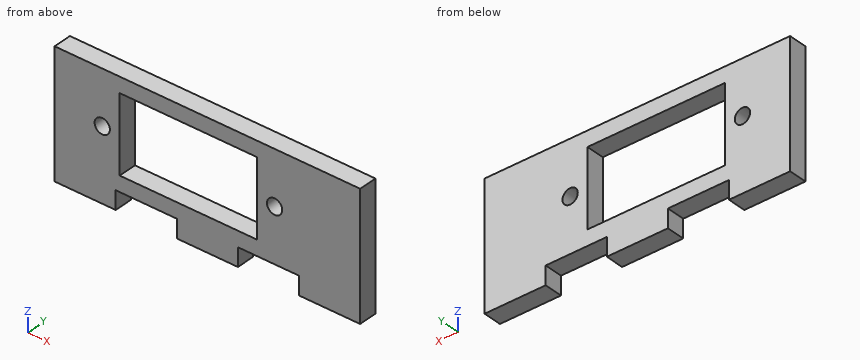
from build123d import *

# Parameters (mm, degrees)
CROQUIS1_R              = 1.25
CROQUIS1_W              = 22.5
CROQUIS1_H              = 12.5
CROQUIS1_W_2            = 10
CROQUIS1_H_2            = 3
SALIENTE_EXTRUIR1_DEPTH = 3


with BuildPart() as part:
    # Croquis1 → Saliente-Extruir1 (new body)
    # profile 1 of 4: a face of its own
    with BuildSketch(Plane(origin=(0, 0, 0), x_dir=(1, 0, 0), z_dir=(0, 1, 0))):
        Polygon((-25, 8.75), (-25, -8.75), (25, -8.75), (25, 8.75), (15, 8.75), (5, 8.75), (-5, 8.75), (-15, 8.75), align=None)
        with Locations(Location((-17.2, 0, 0), (0, 0, 270))):
            Circle(CROQUIS1_R, mode=Mode.SUBTRACT)
        with Locations((-3.1, 0)):
            Rectangle(CROQUIS1_W, CROQUIS1_H, mode=Mode.SUBTRACT)
        with Locations(Location((11, 0, 0), (0, 0, 270))):
            Circle(CROQUIS1_R, mode=Mode.SUBTRACT)
    # profile 2 of 4: a face of its own
    with BuildSketch(Plane(origin=(0, 0, 0), x_dir=(1, 0, 0), z_dir=(0, 1, 0))):
        with Locations((-20, 10.25)):
            Rectangle(CROQUIS1_W_2, CROQUIS1_H_2)
    # profile 3 of 4: a face of its own
    with BuildSketch(Plane(origin=(0, 0, 0), x_dir=(1, 0, 0), z_dir=(0, 1, 0))):
        with Locations((20, 10.25)):
            Rectangle(CROQUIS1_W_2, CROQUIS1_H_2)
    # profile 4 of 4: a face of its own
    with BuildSketch(Plane(origin=(0, 0, 0), x_dir=(1, 0, 0), z_dir=(0, 1, 0))):
        with Locations((0, 10.25)):
            Rectangle(CROQUIS1_W_2, CROQUIS1_H_2)
    extrude(amount=SALIENTE_EXTRUIR1_DEPTH)


solid = part.part
Here's how the part is built. I have some questions about the finished solid (model axes, mm). Round coordinates to 2 decimals unless told otherwise and drop trailing zeros. Write each loop counter-clockwise with the first axis right and the second up, starting at its lowest first coordinate (ties: lowest second). Pieces come first, ordered by that corner, then holes.
1. Suppose I cut it at C-C (z = 0). List the corners of the cut face in (x, y) for me, and give its area (3 significant figures).
2. Suppose I cut it at A-A (x = 11). List the corners of the cut face in (y, z) for me, and give its area (3 significant figures).
3. Suppose I cut it at B-B (y = 1.2). List the corners of the cut face in (x, z) for me.
4. Will these pins go through, and if not, where does the flat tip stop? pin 1 Ø1 at (x, z) = (-16, 1) entering from -Y; pin 2 Ø1.5 at (x, y) = (-9.5, 1.5) entering from -Z; pin 3 Ø2 at (x, z) = (11, 0) entering from +Y.
5. I need wall thicknesses on L1, parallel to X at y = 1.1, z = 0; L2, parallel to X at y = 1.2, z = 2.5; L3, parallel to Z at x = -0.5, y = 0.65. Which ranges of each line are inside material? Lowest first, please.
6. Suppose I cut it at D-D (x = -17.2). List the corners of the cut face in (y, z) for me, and give its area (3 significant figures).
Answer sheet:
1. outline: (-25, 0) - (-18.45, 0) - (-18.45, 3) - (-25, 3) - close; (-15.95, 0) - (-14.35, 0) - (-14.35, 3) - (-15.95, 3) - close; (8.15, 0) - (9.75, 0) - (9.75, 3) - (8.15, 3) - close; (12.25, 0) - (25, 0) - (25, 3) - (12.25, 3) - close
1. area: 67.5 mm2
2. outline: (0, -8.75) - (3, -8.75) - (3, -1.25) - (0, -1.25) - close; (0, 1.25) - (3, 1.25) - (3, 8.75) - (0, 8.75) - close
2. area: 45.0 mm2
3. outline: (-25, -11.75) - (-15, -11.75) - (-15, -8.75) - (-5, -8.75) - (-5, -11.75) - (5, -11.75) - (5, -8.75) - (15, -8.75) - (15, -11.75) - (25, -11.75) - (25, 8.75) - (-25, 8.75) - close; hole circle Ø2.5 at (-17.2, 0); hole (-14.35, -6.25) - (8.15, -6.25) - (8.15, 6.25) - (-14.35, 6.25) - close; hole circle Ø2.5 at (11, 0)
4. pin 1: stops at y = 0
4. pin 2: stops at z = -8.75
4. pin 3: passes through
5. L1: x = -25 to -18.45, -15.95 to -14.35, 8.15 to 9.75, 12.25 to 25
5. L2: x = -25 to -14.35, 8.15 to 25
5. L3: z = -11.75 to -6.25, 6.25 to 8.75
6. outline: (0, -11.75) - (3, -11.75) - (3, -1.25) - (0, -1.25) - close; (0, 1.25) - (3, 1.25) - (3, 8.75) - (0, 8.75) - close
6. area: 54.0 mm2
